```python
from build123d import *

# Parameters (mm, degrees)
SKETCH_1_R          = 3.7
EXTRUDE_1_DEPTH     = 5
CUT_EXTRUDE_1_DEPTH = 3
SKETCH_3_R          = 2
CUT_EXTRUDE_2_DEPTH = 2


with BuildPart() as part:
    # 草图1 → 凸台-拉伸1 (new body)
    with BuildSketch(Plane.XY):
        Circle(SKETCH_1_R)
    extrude(amount=EXTRUDE_1_DEPTH)

    # 草图2 → 切除-拉伸1 (cut)
    with BuildSketch(Plane.XY.offset(5)):
        with BuildLine():
            Line((-1.636863732, 2.595563457), (1.646192649, 2.595563457))
            ThreePointArc((1.646192649, 2.595563457), (2.35329943, 2.302670238), (2.646192649, 1.595563457))
            Line((2.646192649, 1.595563457), (2.646192649, -1.586051907))
            ThreePointArc((2.646192649, -1.586051907), (2.35329943, -2.293158688), (1.646192649, -2.586051907))
            Line((1.646192649, -2.586051907), (-1.636863732, -2.586051907))
            ThreePointArc((-1.636863732, -2.586051907), (-2.343970513, -2.293158688), (-2.636863732, -1.586051907))
            Line((-2.636863732, -1.586051907), (-2.636863732, 1.595563457))
            ThreePointArc((-2.636863732, 1.595563457), (-2.343970513, 2.302670238), (-1.636863732, 2.595563457))
        make_face()
    extrude(amount=-CUT_EXTRUDE_1_DEPTH, mode=Mode.SUBTRACT)

    # 草图3 → 切除-拉伸2 (cut)
    with BuildSketch(Plane.XY.offset(2)):
        Circle(SKETCH_3_R)
    extrude(amount=-CUT_EXTRUDE_2_DEPTH, mode=Mode.SUBTRACT)


solid = part.part
```
Check sheet for the modelled part. Datum: model origin and axes. Units: mm. A direction names the side the tool comes from. Give positions to 0.01 mm unless a question says otherwise; leave off trailing zeros. Order: outer loops, then holes, each group sorted by start corner. A loop starts at its lowest first (then second) coordinate and runs counter-clockwise, first axis right, second up. Notation, with made-up numbers: M 34,72 L 78,72 A26 cw 78,93 Z; hole C 42,-26 d10. An arc over 180 degrees is marked long. Answer in a Markdown table with one row per item. Add a question column.
Q1. Thickness scan on L1, parallel to Y at x = 0, z = 1.65; L2, parallel to Z at x = 2.5, y = -1.5; L3, parallel to X at y = 0.5, z = 2.6. Record the ranges inside material, lowest first.
Q2. Sectioned sample at B-B, the plane x = 0. Record the boundary of the cut face in (y, z).
Q3. Sectioned sample at C-C, the plane z = 4.6. Record the boundary of the cut face in (x, y).
Q4. Sectioned sample at D-D, the plane y = -2.25. Record the boundary of the cut face in (x, z), and give its area (3 significant figures).
Q5. Sectioned sample at A-A, the plane y = 0. Record the boundary of the cut face in (x, z), and give its area (3 significant figures).
Q6. Access from +Z, -Z, +X, -X, +Y, -Y to the whole of each face (thin tool, end or side, straight path). Record for faces 1 (the flat face through (0, -2.586, 4)), 2 (the cylindrical face through (0, -2, 1)).
Q7. Release check for a two-part mould opening along X. For faces 3 (the cylindrical face through (2.361, -2.285, 3.521)), 4 (the cylindrical face through (-0.802, -3.612, 2.465)), 5 (the flat face through (3, 0, 5)) record: released by +X, released by -X, zero draft, split by the parting line, or undercut.
Q8. Gauge pin test, flat ends, axial feed: pin 1 Ø2.5 at (x, y) = (1, -1) entering from +Z; pin 2 Ø3 at (x, y) = (0, 0) entering from +Z. Record the tip position at first contact, or that the pin passes through.
Verdict:
| question | item | result |
|---|---|---|
| 1 | L1 | -3.7 to -2, 2 to 3.7 |
| 1 | L2 | 0 to 2 |
| 1 | L3 | -3.67 to -2.64, 2.65 to 3.67 |
| 2 | outline | M -3.7,0 L -2,0 L -2,2 L -2.59,2 L -2.59,5 L -3.7,5 Z; M 2,0 L 3.7,0 L 3.7,5 L 2.6,5 L 2.6,2 L 2,2 Z |
| 3 | outline | C 0,0 d7.4; hole M -2.64,-1.59 A1 ccw -1.64,-2.59 L 1.65,-2.59 A1 ccw 2.65,-1.59 L 2.65,1.6 A1 ccw 1.65,2.6 L -1.64,2.6 A1 ccw -2.64,1.6 Z |
| 4 | outline | M -2.94,0 L 2.94,0 L 2.94,5 L 2.39,5 L 2.39,2 L -2.38,2 L -2.38,5 L -2.94,5 Z |
| 4 | area | 15.0 mm² |
| 5 | outline | M -3.7,0 L -2,0 L -2,2 L -2.64,2 L -2.64,5 L -3.7,5 Z; M 2,0 L 3.7,0 L 3.7,5 L 2.65,5 L 2.65,2 L 2,2 Z |
| 5 | area | 13.2 mm² |
| 6 | face 1 | +Z |
| 6 | face 2 | +Z, -Z |
| 7 | face 3 | undercut |
| 7 | face 4 | split by the parting line |
| 7 | face 5 | zero draft |
| 8 | pin 1 | z = 2 |
| 8 | pin 2 | through |
